Check sheet for the modelled part. Datum: model origin and axes. Units: mm. Give positions to 0.01 mm unless a question says otherwise; leave off trailing zeros. Loops run counter-clockwise (first coordinate to the right, second up) from the corner with the lowest first, then second, coordinate; pieces in that order, holes last. Notation, with made-up numbers: (41.5, 32.5) -> (51.5, 32.5) arc R11 cw to (51.5, 40.5) -> close; hole circle Ø4 at (31.25, -10). An arc over 180 degrees is marked (long way). Write each question's results on one line, items separated by ' | '. Start each with the question number.
Item 1: Gauge pin test, flat ends, axial feed: pin 1 Ø3 at (y, z) = (431.5, -13) entering from -X; pin 2 Ø1.5 at (x, y) = (-25, 81.5) entering from -Z; pin 3 Ø6 at (y, z) = (486.5, -24) entering from -X. Record the tip position at first contact, or that the pin passes through.
Item 2: Cross-section at B-B on x = -20. Enter the section's corners in (y, z).
Item 3: Scan lines: line 1 along X through (y, z) = (353, -29); line 2 along X through (y, z) = (51.5, -10); line 3 along Z through (x, y) = (-35.5, 419). Record each from-to range of solid material in increasing order.
Item 4: Cross-section at C-C on y = 534.5. Enter the section's corners in (x, z).
Item 5: Cross-section at A-A on z = -21. Enter the section's corners in (x, y), then the cut area to 3 significant figures.
Autodesk Inventor part; units mm, degrees
ref_plane "YZ Plane" through (0, 0, 0) normal (1, 0, 0) x (0, 1, 0)
ref_plane "XZ Plane" through (0, 0, 0) normal (0, 1, 0) x (-1, 0, 0)
ref_plane "XY Plane" through (0, 0, 0) normal (0, 0, 1) x (1, 0, 0)
sketch "Esboço1" plane through (0, 0, 0) normal (0, 1, 0) x (-1, 0, 0)
  line L0 (0, 0) -> (40, 0)
  line L1 (0, -40) -> (0, 0)
  line L2 (0, -40) -> (40, 0)
extrude "Extrusão1" add sketch "Esboço1" along normal blind 700
sketch "Esboço2" plane through (-40, 0, 0) normal (-0.7071, 0, -0.7071) x (-0.7071, 0, 0.7071)
  line L0 (0, 700) -> (-28.2843, 700)
  line L1 (-28.2843, 700) -> (-28.2843, 600)
  line L2 (-28.2843, 0) -> (-28.2843, 700)
  line L3 (-28.2843, 600) -> (-6.7843, 600)
  line L4 (-6.7843, 600) -> (-28.2843, 600)
  line L5 (-28.2843, 600) -> (-49.7843, 600)
  dimension "d4" = 100
  dimension "d5" = 21.5
  dimension "d6" = 21.5
hole "Furo1" at (-35.2028, 600, -4.7972) at (-4.7972, 600, -35.2028) direction (0.7071, 0, 0.7071) diameter 3 end through all
sketch "Esboço3" plane through (-40, 0, 0) normal (-0.7071, 0, -0.7071) x (-0.7071, 0, 0.7071)
  circle A0 centre (-6.7843, 600) radius 1.5
  line L0 (-6.7843, 600) -> (-6.7843, 132)
  circle A1 centre (-49.7843, 600) radius 1.5
  line L1 (-49.7843, 600) -> (-49.7843, 132)
  point P0 (-28.2843, 0)
  dimension "d14" = 468
  dimension "d15" = 468
hole "Furo2" at (-35.2028, 132, -4.7972) at (-4.7972, 132, -35.2028) direction (0.7071, 0, 0.7071) diameter 3 end through all
sketch "Esboço4" plane through (-40, 0, 0) normal (-0.7071, 0, -0.7071) x (-0.7071, 0, 0.7071)
  circle A0 centre (-49.7843, 600) radius 1.5
  line L0 (-49.7843, 600) -> (-49.7843, 633)
  point P0 (-28.2843, 0)
  point P1 (-6.7843, 633)
  dimension "d23" = 33
hole "Furo3" at (-4.7972, 633, -35.2028) at (-35.2028, 633, -4.7972) direction (0.7071, 0, 0.7071) diameter 3 end through all
properties part number "coluna" material "Madeira (Bétula)"
Answer sheet:
1) pin 1: stops at x = -28.5 | pin 2: stops at z = -15.75 | pin 3: stops at x = -19
2) outline: (0, -20) -> (700, -20) -> (700, 0) -> (0, 0) -> close
3) line 1: x = -11 to 0 | line 2: x = -30 to 0 | line 3: z = -4.5 to 0
4) outline: (-40, 0) -> (0, -40) -> (0, 0) -> close
5) outline: (-19, 0) -> (0, 0) -> (0, 700) -> (-19, 700) -> close | area: 13,300 mm²
